Autodesk Inventor part; units mm, degrees
ref_plane "Work Plane1" through (0, 0, 0) normal (0, 0, 1) x (1, 0, 0)
ref_plane "Work Plane2" through (0, -43.3, 2) normal (-1, 0, 0) x (0, 0, 1)
ref_plane "YZ Plane" through (0, 0, 0) normal (1, 0, 0) x (0, 1, 0)
ref_plane "Work Plane1" through (0, 0, 0) normal (0, 0, 1) x (1, 0, 0)
sketch "Sketch1" plane through (0, 0, 0) normal (0, 0, 1) x (1, 0, 0)
  line L0 (-12.7, 12) -> (-9.2, 12) construction
  line L1 (-12.7, 12) -> (-17.8, 6) construction
  line L2 (-17.8, 6) -> (-17.8, -32.6) construction
  line L3 (-17.8, -32.6) -> (-12.7, -38.6) construction
  line L4 (-12.7, -38.6) -> (12.7, -38.6) construction
  line L5 (12.7, -38.6) -> (17.8, -32.6) construction
  line L6 (17.8, -32.6) -> (17.8, 6) construction
  line L7 (17.8, 6) -> (12.7, 12) construction
  line L8 (9.2, 12) -> (12.7, 12) construction
  arc A0 (12.2, 9) -> (9.2, 12) centre (9.2, 9) ccw construction
  line L9 (12.2, -30) -> (12.2, 9) construction
  arc A1 (9.2, -33) -> (12.2, -30) centre (9.2, -30) ccw construction
  line L10 (-9.2, -33) -> (9.2, -33) construction
  arc A2 (-12.2, -30) -> (-9.2, -33) centre (-9.2, -30) ccw construction
  line L11 (-12.2, 9) -> (-12.2, -30) construction
  arc A3 (-9.2, 12) -> (-12.2, 9) centre (-9.2, 9) ccw construction
  circle A4 centre (-15, 4.5) radius 1.35 construction
  circle A5 centre (-15, -12.5) radius 1.35 construction
  circle A6 centre (-8.5, -35.8) radius 1.35 construction
  circle A7 centre (15, 4.5) radius 1.35 construction
  circle A8 centre (15, -12.5) radius 1.35 construction
  circle A9 centre (8.5, -35.8) radius 1.35 construction
  circle A10 centre (-15, -29.5) radius 1.35 construction
  circle A11 centre (15, -29.5) radius 1.35 construction
  line L12 (-15, -12.5) -> (-12.5, -12.5) construction
  line L13 (-12.5, -12.5) -> (-12.5, -9.5) construction
  line L14 (-12.5, -9.5) -> (-15, -9.5) construction
  line L15 (-15, -9.5) -> (-15, -12.5) construction
  line L16 (15, -12.5) -> (12.5, -12.5) construction
  line L17 (12.5, -12.5) -> (12.5, -9.5) construction
  line L18 (12.5, -9.5) -> (15, -9.5) construction
  line L19 (15, -9.5) -> (15, -12.5) construction
  line L20 (-8.5, -35.8) -> (-12.5, -35.8) construction
  line L21 (-12.5, -35.8) -> (-12.5, -33.3) construction
  line L22 (-12.5, -33.3) -> (-8.5, -33.3) construction
  line L23 (-8.5, -33.3) -> (-8.5, -35.8) construction
  line L24 (8.5, -35.8) -> (12.5, -35.8) construction
  line L25 (12.5, -35.8) -> (12.5, -33.3) construction
  line L26 (12.5, -33.3) -> (8.5, -33.3) construction
  line L27 (8.5, -33.3) -> (8.5, -35.8) construction
  line L28 (-12.5, -9.5) -> (-22.5, -9.5)
  line L29 (-22.5, -9.5) -> (-22.5, -33.3)
  line L30 (-22.5, -33.3) -> (-12.5, -33.3)
  line L31 (-12.5, -33.3) -> (-12.5, -9.5)
  line L32 (12.5, -9.5) -> (22.5, -9.5)
  line L33 (22.5, -9.5) -> (22.5, -33.3)
  line L34 (22.5, -33.3) -> (12.5, -33.3)
  line L35 (12.5, -33.3) -> (12.5, -9.5)
  line L36 (-22.5, -33.3) -> (22.5, -33.3)
  line L37 (22.5, -33.3) -> (22.5, -43.3)
  line L38 (22.5, -43.3) -> (-22.5, -43.3)
  line L39 (-22.5, -43.3) -> (-22.5, -33.3)
  circle A12 centre (-15, -12.5) radius 1.5
  circle A13 centre (-15, -29.5) radius 1.5
  circle A14 centre (-8.5, -35.8) radius 1.5
  circle A15 centre (8.5, -35.8) radius 1.5
  circle A16 centre (15, -29.5) radius 1.5
  circle A17 centre (15, -12.5) radius 1.5
  point P0 (0, 0)
  dimension "d0" = 2.5
  dimension "d1" = 3
  dimension "d2" = 2.5
  dimension "d3" = 3
  dimension "d4" = 4
  dimension "d5" = 2.5
  dimension "d6" = 4
  dimension "d7" = 2.5
  dimension "d9" = 10
  dimension "d10" = 10
  dimension "d11" = 10
  dimension "d12" = 3
  dimension "d13" = 3
  dimension "d14" = 3
  dimension "d15" = 3
  dimension "d16" = 3
  dimension "d17" = 3
extrude "Extrusion1" add sketch "Sketch1" along normal blind 2
sketch "Sketch2" plane through (-22.5, -43.3, 0) normal (0, -1, 0) x (1, 0, 0)
  line L0 (0, 0) -> (45, 0)
  line L1 (45, 0) -> (45, 2)
  line L2 (0, 2) -> (45, 2)
  line L3 (0, 0) -> (0, 2)
  line L4 (0, 0) -> (45, 0)
  line L5 (45, 0) -> (45, -20)
  line L6 (45, -20) -> (0, -20)
  line L7 (0, -20) -> (0, 0)
  point P0 (22.5, 0)
  dimension "d20" = 20
extrude "Extrusion2" add sketch "Sketch2" against normal blind 4
ref_plane "Work Plane2" through (0, -43.3, 2) normal (-1, 0, 0) x (0, 0, 1)
sketch "Sketch3" plane through (-22.5, -43.3, 2) normal (-1, 0, 0) x (0, 0, 1)
  line L0 (0, 33.8) -> (0, 0)
  line L1 (-2, 33.8) -> (0, 33.8)
  line L2 (-2, 33.8) -> (-2, 4)
  line L3 (-22, 4) -> (-2, 4)
  line L4 (-22, 0) -> (-22, 4)
  line L5 (-22, 0) -> (0, 0)
  line L6 (-2, 33.8) -> (-2, 4)
  line L7 (-2, 4) -> (-22, 4)
  line L8 (-22, 4) -> (-22, 33.8)
  line L9 (-22, 33.8) -> (-2, 33.8)
  line L10 (-2, 33.8) -> (-2, 4)
  point P0 (-2, 43.3)
extrude "Extrusion3" add sketch "Sketch3" against normal blind 4
mirror "Mirror1" about plane through (0, -43.3, 2) normal (-1, 0, 0) of "Extrusion3"
sketch "Sketch4" plane through (0, 0, 2) normal (0, 0, 1) x (1, 0, 0)
  line L0 (22.5, -9.5) -> (12.5, -9.5)
  line L1 (12.5, -9.5) -> (12.5, -33.3)
  line L2 (12.5, -33.3) -> (-12.5, -33.3)
  line L3 (-12.5, -33.3) -> (-12.5, -9.5)
  line L4 (-12.5, -9.5) -> (-22.5, -9.5)
  line L5 (-22.5, -9.5) -> (-22.5, -43.3)
  line L6 (-22.5, -43.3) -> (22.5, -43.3)
  line L7 (22.5, -43.3) -> (22.5, -9.5)
  circle A0 centre (8.5, -35.8) radius 1.5
  circle A1 centre (-8.5, -35.8) radius 1.5
  circle A2 centre (15, -12.5) radius 1.5
  circle A3 centre (15, -29.5) radius 1.5
  circle A4 centre (-15, -29.5) radius 1.5
  circle A5 centre (-15, -12.5) radius 1.5
  circle A6 centre (8.5, -35.8) radius 2.5
  circle A7 centre (15, -29.5) radius 1.5
  circle A8 centre (15, -29.5) radius 2.5
  circle A9 centre (15, -12.5) radius 2.5
  circle A10 centre (-8.5, -35.8) radius 2.5
  circle A11 centre (-15, -29.5) radius 1.5
  circle A12 centre (-15, -29.5) radius 2.5
  circle A13 centre (-15, -12.5) radius 2.5
  point P0 (0, 0)
  dimension "d25" = 5
  dimension "d26" = 5
  dimension "d27" = 5
  dimension "d28" = 5
  dimension "d29" = 5
  dimension "d30" = 5
extrude "Extrusion4" add sketch "Sketch4" along normal blind 2 contours L7 L6 L5 L4 L3 L2 L1 L0
sketch "Sketch5" plane through (-22.5, -43.3, -20) normal (0, -1, 0) x (1, 0, 0)
  line L0 (0, 0) -> (0, 24) construction
  line L1 (0, 0) -> (45, 0) construction
  line L2 (45, 0) -> (45, 24) construction
  line L3 (0, 24) -> (45, 24) construction
  line L4 (0, 24) -> (15, 24) construction
  line L5 (15, 24) -> (15, 9) construction
  line L6 (15, 9) -> (0, 9) construction
  line L7 (0, 9) -> (0, 24) construction
  line L8 (15, 9) -> (30, 9) construction
  circle A0 centre (15, 9) radius 1.5
  circle A1 centre (30, 9) radius 1.5
  point P0 (22.5, 20)
  dimension "d33" = 15
  dimension "d34" = 15
  dimension "d35" = 15
  dimension "d36" = 3
  dimension "d37" = 3
extrude "Extrusion5" cut sketch "Sketch5" against normal through all
sketch "Sketch6" plane through (-22.5, -39.3, 0) normal (0, 1, 0) x (1, 0, 0)
  circle A0 centre (15, 11) radius 1.5
  circle A1 centre (30, 11) radius 1.5
  line L0 (41, 0) -> (41, 20)
  line L1 (41, 20) -> (4, 20)
  line L2 (4, 20) -> (4, 0)
  line L3 (41, 0) -> (4, 0)
  line L4 (15, 11) -> (17.6, 11)
  line L5 (17.6, 9.4989) -> (15, 7.9978)
  line L6 (15, 7.9978) -> (12.4, 9.4989)
  line L7 (12.4, 9.4989) -> (12.4, 12.5011)
  line L8 (12.4, 12.5011) -> (15, 14.0022)
  line L9 (15, 14.0022) -> (17.6, 12.5011)
  line L10 (17.6, 12.5011) -> (17.6, 9.4989)
  line L11 (30, 11) -> (32.6, 11)
  line L12 (32.6, 9.4989) -> (30, 7.9978)
  line L13 (30, 7.9978) -> (27.4, 9.4989)
  line L14 (27.4, 9.4989) -> (27.4, 12.5011)
  line L15 (27.4, 12.5011) -> (30, 14.0022)
  line L16 (30, 14.0022) -> (32.6, 12.5011)
  line L17 (32.6, 12.5011) -> (32.6, 9.4989)
  point P0 (22.5, 0)
  dimension "d40" = 2.6
  dimension "d41" = 2.6
extrude "Extrusion6" cut sketch "Sketch6" against normal blind 2 contours L10 L5 L6 L7 L8 L9 | L17 L12 L13 L14 L15 L16
sketch "Sketch7" plane through (-22.5, -43.3, -20) normal (-1, 0, 0) x (0, 0, 1)
  line L0 (0, 33.8) -> (24, 33.8) construction
  line L1 (0, 0) -> (0, 33.8) construction
  line L2 (0, 0) -> (24, 0) construction
  line L3 (24, 33.8) -> (24, 0) construction
  line L4 (0, 33.8) -> (10, 33.8) construction
  line L5 (10, 33.8) -> (10, 28.8) construction
  line L6 (10, 28.8) -> (0, 28.8) construction
  line L7 (0, 28.8) -> (0, 33.8) construction
  line L8 (0, 0) -> (0, 33.8) construction
  line L9 (0, 0) -> (9, 0) construction
  line L10 (9, 0) -> (9, 12) construction
  line L11 (9, 12) -> (0, 12) construction
  line L12 (0, 12) -> (0, 0) construction
  line L13 (9, 12) -> (9, 27) construction
  circle A0 centre (9, 27) radius 1.5
  circle A1 centre (9, 12) radius 1.5
  point P0 (20, 43.3)
  dimension "d44" = 10
  dimension "d45" = 5
  dimension "d46" = 9
  dimension "d47" = 12
  dimension "d48" = 15
  dimension "d49" = 3
  dimension "d50" = 3
extrude "Extrusion7" cut sketch "Sketch7" against normal through all
sketch "Sketch8" plane through (-18.5, -43.3, 2) normal (1, 0, 0) x (0, 0, -1)
  circle A0 centre (13, 27) radius 1.5 construction
  circle A1 centre (13, 12) radius 1.5 construction
  line L0 (22, 4) -> (2, 4) construction
  line L1 (22, 4) -> (22, 33.8) construction
  line L2 (22, 33.8) -> (2, 33.8) construction
  line L3 (2, 4) -> (2, 33.8) construction
  line L4 (13, 12) -> (13, 14.6) construction
  line L5 (14.5011, 14.6) -> (16.0022, 12)
  line L6 (16.0022, 12) -> (14.5011, 9.4)
  line L7 (14.5011, 9.4) -> (11.4989, 9.4)
  line L8 (11.4989, 9.4) -> (9.9978, 12)
  line L9 (9.9978, 12) -> (11.4989, 14.6)
  line L10 (11.4989, 14.6) -> (14.5011, 14.6)
  circle A2 centre (13, 27) radius 1.5
  line L11 (13, 27) -> (13, 29.6)
  line L12 (14.5011, 29.6) -> (16.0022, 27)
  line L13 (16.0022, 27) -> (14.5011, 24.4)
  line L14 (14.5011, 24.4) -> (11.4989, 24.4)
  line L15 (11.4989, 24.4) -> (9.9978, 27)
  line L16 (9.9978, 27) -> (11.4989, 29.6)
  line L17 (11.4989, 29.6) -> (14.5011, 29.6)
  point P0 (2, 43.3)
  dimension "d53" = 2.6
  dimension "d54" = 2.6
extrude "Extrusion8" cut sketch "Sketch8" against normal blind 2
mirror "Mirror2" about plane through (0, -43.3, 2) normal (-1, 0, 0) of "Extrusion8"
properties part number "april_tag"
Can you work these out from the model? Positions are in its coordinate system, mm. A direction names the side the tool comes from. Round coordinates to 2 decimals unless told otherwise and drop trailing zeros. Order: outer loops, then holes, each group sorted by start corner. A loop starts at its lowest first (then second) coordinate and runs counter-clockwise, first axis right, second up. Notation, with made-up numbers: (87.5, 68.25) -> (146.5, 68.25) arc R27 cw to (146.5, 105.25) -> close; hole circle Ø9 at (84.25, -33.75). An arc over 180 degrees is marked (long way). Return JSON: item names as keys, results as strings. Group by question number.
1. Will these pins go through, and if not, where does the flat tip stop? pin 1 (12 mm diameter, centred on x = 3.5, z = -4.5, fed in from +Y); pin 2 (2.5 mm diameter, centred on y = -31.3, z = -11, fed in from +X); pin 3 (1.5 mm diameter, centred on x = -12.5, y = -17.5, fed in from -Z); pin 4 (2.5 mm diameter, centred on x = 15.5, y = -30.5, fed in from +Z).
2. If we section it at C-C, the plane x = -20: Write out the boundary of the cut face in (y, z).
3. If we section it at D-D, the plane y = -17: Write out the boundary of the cut face in (x, z).
4. I need wall thicknesses on line 1 (X direction, y = -42.7, z = -11); line 2 (Y direction, x = -21.4, z = -11); line 3 (X direction, y = -34, z = -10.75). Which ranges of each line are inside material? Lowest first, please. Write a range as [from, to].
5. If we section it at A-A, the plane y = -21: Write out the boundary of the cut face in (x, z).
6. If we section it at B-B, the plane x = 15: Write out the boundary of the cut face in (y, z), then the cut area to 3 significant figures.
7. Which directions (+Z, -Z, +X, -X, +Y, -Y) give clear straight access to the entire face, cutting with the end or side of a thin tool? Please do faces 4 (the face through (-6.18, -40.29, -8.76)), 5 (the face through (-7, -37, 2)), 6 (the face through (20, -9.5, -8)), 7 (the face through (-19.49, -29.98, -13.24)), 8 (the face through (0, -39.3, -10)).
8. We'd pull the mould along Z, two halves only. Please class faces 1 (the face through (-20, -9.5, -8)), 2 (the face through (-21.514, -14.813, -11.195)), 3 (the face through (10, -37, 2)): released by +Z, released by -Z, zero draft, split by the parting line, or undercut.
Output values:
{
 "1": {"pin 1": "y = -33.3", "pin 2": "through", "pin 3": "z = 0", "pin 4": "z = 2"},
 "2": {"outline": "(-43.3, -20) -> (-9.5, -20) -> (-9.5, 4) -> (-43.3, 4) -> close; hole (-33.9, -12.5) -> (-31.3, -14) -> (-28.7, -12.5) -> (-28.7, -9.5) -> (-31.3, -8) -> (-33.9, -9.5) -> close; hole (-18.9, -12.5) -> (-16.3, -14) -> (-13.7, -12.5) -> (-13.7, -9.5) -> (-16.3, -8) -> (-18.9, -9.5) -> close"},
 "3": {"outline": "(-22.5, -20) -> (-18.5, -20) -> (-18.5, -13.6) -> (-20.5, -13.6) -> (-20.5, -12.33) -> (-22.5, -12.33) -> close; (-22.5, -9.67) -> (-20.5, -9.67) -> (-20.5, -8.4) -> (-18.5, -8.4) -> (-18.5, 0) -> (-12.5, 0) -> (-12.5, 4) -> (-22.5, 4) -> close; (12.5, 0) -> (18.5, 0) -> (18.5, -8.4) -> (20.5, -8.4) -> (20.5, -9.67) -> (22.5, -9.67) -> (22.5, 4) -> (12.5, 4) -> close; (18.5, -20) -> (22.5, -20) -> (22.5, -12.33) -> (20.5, -12.33) -> (20.5, -13.6) -> (18.5, -13.6) -> close"},
 "4": {"line 1": "[-22.5, -9], [-6, 6], [9, 22.5]", "line 2": "[-43.3, -32.8], [-29.8, -17.8], [-14.8, -9.5]", "line 3": "[-22.5, -18.5], [18.5, 22.5]"},
 "5": {"outline": "(-22.5, -20) -> (-18.5, -20) -> (-18.5, 0) -> (-12.5, 0) -> (-12.5, 4) -> (-22.5, 4) -> close; (12.5, 0) -> (18.5, 0) -> (18.5, -20) -> (22.5, -20) -> (22.5, 4) -> (12.5, 4) -> close"},
 "6": {"outline": "(-43.3, -20) -> (-39.3, -20) -> (-39.3, 0) -> (-31, 0) -> (-31, 2) -> (-32, 2) -> (-32, 4) -> (-43.3, 4) -> close; (-28, 0) -> (-14, 0) -> (-14, 2) -> (-15, 2) -> (-15, 4) -> (-27, 4) -> (-27, 2) -> (-28, 2) -> close; (-11, 0) -> (-9.5, 0) -> (-9.5, 4) -> (-10, 4) -> (-10, 2) -> (-11, 2) -> close", "area": "183 mm²"},
 "7": {"face 4": "+Y", "face 5": "+Z", "face 6": "+Z, -Z, +X, -X, +Y", "face 7": "none", "face 8": "-Z, +Y"},
 "8": {"face 1": "zero draft", "face 2": "undercut", "face 3": "released by +Z"}
}
